Source: CAD feature listing. Evaluate the final solid. Frame: model axes, mm. Round coordinates to 2 decimals unless told otherwise and drop trailing zeros. Write each loop counter-clockwise with the first axis right and the second up, starting at its lowest first coordinate (ties: lowest second). Pieces come first, ordered by that corner, then holes. Notation, with made-up numbers: M 15.5,44.25 L 32.5,44.25 A27 ccw 32.5,64.25 Z; hole C -40,48 d10. An arc over 180 degrees is marked long. Use a Markdown table: item, result.
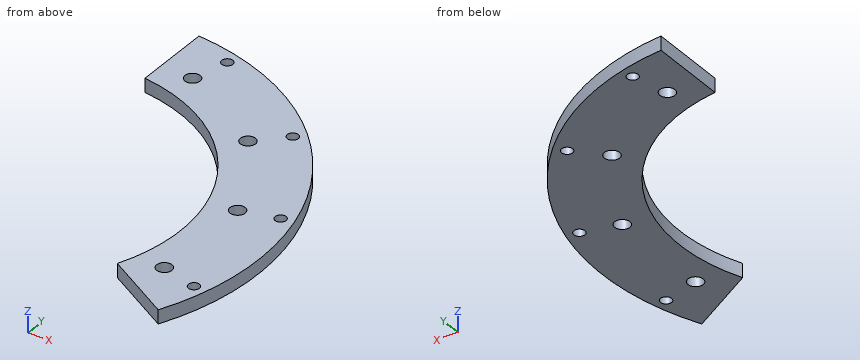
```python
from build123d import *

# Parameters (mm, degrees)
BOSS_EXTRU_1_DEPTH = 4
SKETCH2_R          = 1.6
SKETCH2_R_2        = 2.2
CUT_EXTRUDE1_DEPTH = 105.004154725
CIRPATTERN1_COUNT  = 12


with BuildPart() as part:
    # Esquisse1 → Boss.-Extru.1 (new body)
    with BuildSketch(Plane.XY):
        with BuildLine():
            Line((6, 73.365060485), (6, 50.746526975))
            ThreePointArc((6, 50.746526975), (44.255153019, 25.547826351), (46.94579921, -20.181722835))
            Line((46.94579921, -20.181722835), (66.533866524, -31.490898771))
            ThreePointArc((66.533866524, -31.490898771), (63.749380359, 36.802834183), (6, 73.365060485))
        make_face()
    extrude(amount=BOSS_EXTRU_1_DEPTH)

    # Sketch2 → Cut-Extrude1 (cut, through all)
    with BuildSketch(Plane.XY.offset(4)):
        with Locations((18.117333157, 67.61480784)):
            Circle(SKETCH2_R)
        with Locations((15.316911089, 57.1634904)):
            Circle(SKETCH2_R_2)
    cut_extrude1 = extrude(amount=-CUT_EXTRUDE1_DEPTH, mode=Mode.SUBTRACT)

    # CirPattern1: Cut-Extrude1 ×12 about axis
    cirpattern1_axis = Axis((0, 0, 0), (0, 0, 1))
    for i in range(1, CIRPATTERN1_COUNT):
        add(cut_extrude1.rotate(cirpattern1_axis, i * 360 / CIRPATTERN1_COUNT), mode=Mode.SUBTRACT)


solid = part.part
```
Q1. Section B-B on x = 12. Return loops of the section in (y, z), plus the area to 3 significant figures.
Results are:
| item | result |
|---|---|
| outline | M 49.67,0 L 72.63,0 L 72.63,4 L 49.67,4 Z |
| area | 91.8 mm^2 |
Q2. Line query: L1, parallel to Y at x = 56, z = 3.35; L2, parallel to X at y = 41, z = 0.4; L3, parallel to X at y = 67, z = 1.2. Output: solid intervals per line, ascending.
Results are:
| item | result |
|---|---|
| L1 | -25.41 to -17.18, -13.45 to 13.45, 17.18 to 47.77 |
| L2 | 30.5 to 39.82, 43.88 to 61.13 |
| L3 | 6 to 16.64, 19.59 to 30.49 |
Q3. First-contact query: pin 1 Ø1.5 at (x, z) = (32.5, 1) entering from +Y; pin 2 Ø5.5 at (x, y) = (57.16, -15.32) entering from +Z; pin 3 Ø1 at (x, z) = (53, 2.5) entering from -Y. Flat tips, straight axial feed; report the tip coordinate or a pass-through.
Results are:
| item | result |
|---|---|
| pin 1 | y = 66.41 |
| pin 2 | z = 4 |
| pin 3 | y = -23.97 |
Q4. Section C-C on y = 9.5. Return loops of the section in (x, z), plus the area to 3 significant figures.
Results are:
| item | result |
|---|---|
| outline | M 50.21,0 L 72.99,0 L 72.99,4 L 50.21,4 Z |
| area | 91.1 mm^2 |
Q5. Section A-A on z = 1.2. Give the number of separate pieces and of enclosed holes in the cut face, plus the area to 3 significant figures.
Results are:
| item | result |
|---|---|
| separate pieces | 1 |
| enclosed holes | 8 |
| area | 2,580 mm^2 |
